Could you check a few things on this model? Use its own coordinates, in mm. Face numbers are marked on the shaded views. A direction names the side the tool comes from. Round coordinates to 2 decimals unless told otherwise and drop trailing zeros. Write each loop counter-clockwise with the first axis right and the second up, starting at its lowest first coordinate (ties: lowest second). Pieces come first, ordered by that corner, then holes. Notation, with made-up numbers: (69, 77) - (93, 77) arc R15 cw to (93, 89) - close; hole circle Ø6 at (38.5, 16). An arc over 180 degrees is marked (long way). Put each result on its own line as item: value.
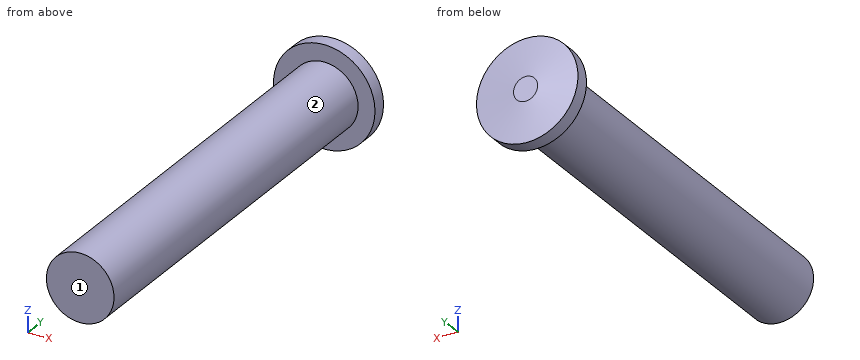
from build123d import *

# Parameters (mm, degrees)
SKETCH1_R           = 3.175
BOSS_EXTRUDE1_DEPTH = 19.05
SKETCH2_R           = 4.7625
BOSS_EXTRUDE2_DEPTH = 1.5875
CHAMFER1_SIZE       = 0.254
CHAMFER1_SIZE2      = 3.632369229


with BuildPart() as part:
    # Sketch1 → Boss-Extrude1 (new body, symmetric)
    with BuildSketch(Plane(origin=(0, 0, 0), x_dir=(1, 0, 0), z_dir=(0, 1, 0))):
        Circle(SKETCH1_R)
    extrude(amount=BOSS_EXTRUDE1_DEPTH, both=True)

    # Sketch2 → Boss-Extrude2 (add)
    with BuildSketch(Plane(origin=(0, 19.05, 0), x_dir=(1, 0, 0), z_dir=(0, 1, 0))):
        Circle(SKETCH2_R)
    extrude(amount=BOSS_EXTRUDE2_DEPTH)

    # Chamfer1
    chamfer1_edges = [part.edges().sort_by_distance(p)[0] for p in [
        (-4.7625, 20.6375, 0),
    ]]
    chamfer1_side = [part.faces().sort_by_distance(p)[0] for p in [
        (-4.7625, 19.84375, 0),
    ]]
    chamfer(chamfer1_edges, length=CHAMFER1_SIZE, length2=CHAMFER1_SIZE2, reference=chamfer1_side[0])


solid = part.part
(1) Please list where these lines run through material, in increasing order: probe 1 along Y at (x, z) = (-0.5, -3.25); probe 2 along Z at (x, y) = (2.25, -13.5); probe 3 along Y at (x, z) = (-4.5, 1). Write a range as from..to.
Values found:
probe 1: y = 19.05..20.49
probe 2: z = -2.24..2.24
probe 3: y = 19.05..20.39
(2) I'm going to push flat-ended pins straight in: pin 1 (4 mm diameter, centred on x = -0.5, z = -3.5, fed in from -Y); pin 2 (1 mm diameter, centred on x = 0, z = -3.5, fed in from +Y); pin 3 (2 mm diameter, centred on x = -1, y = 7.5, fed in from +Z) (3 decimals); pin 4 (1 mm diameter, centred on y = -4, z = 1, fed in from -X). Where does each tip first touch, or does it pass through?
Values found:
pin 1: stops at y = -19.05
pin 2: stops at y = 20.51
pin 3: stops at z = 3.175
pin 4: stops at x = -3.14
(3) Imagine slicing it at C-C, the plane y = 14.5. List the corners of the cut face in (x, z) for me (3 decimals).
Values found:
outline: circle Ø6.35 at (0, 0)
(4) For the marked faces 1 and 2, which set-ups out of +Z, -Z, +X, -X, +Y, -Y let a thin tool reach every point of the face, with its end or its side?
Values found:
face 1: +Z, -Z, +X, -X, -Y
face 2: -Y
